Study the drawing (mm; zero at the part's minimum x, y, z) and answer. Coordinates: 2 decimals unless noted, no trailing zeros. Order: outer loops, then holes, each group sorted by start corner. A loop starts at its lowest first (then second) coordinate and runs counter-clockwise, first axis right, second up.
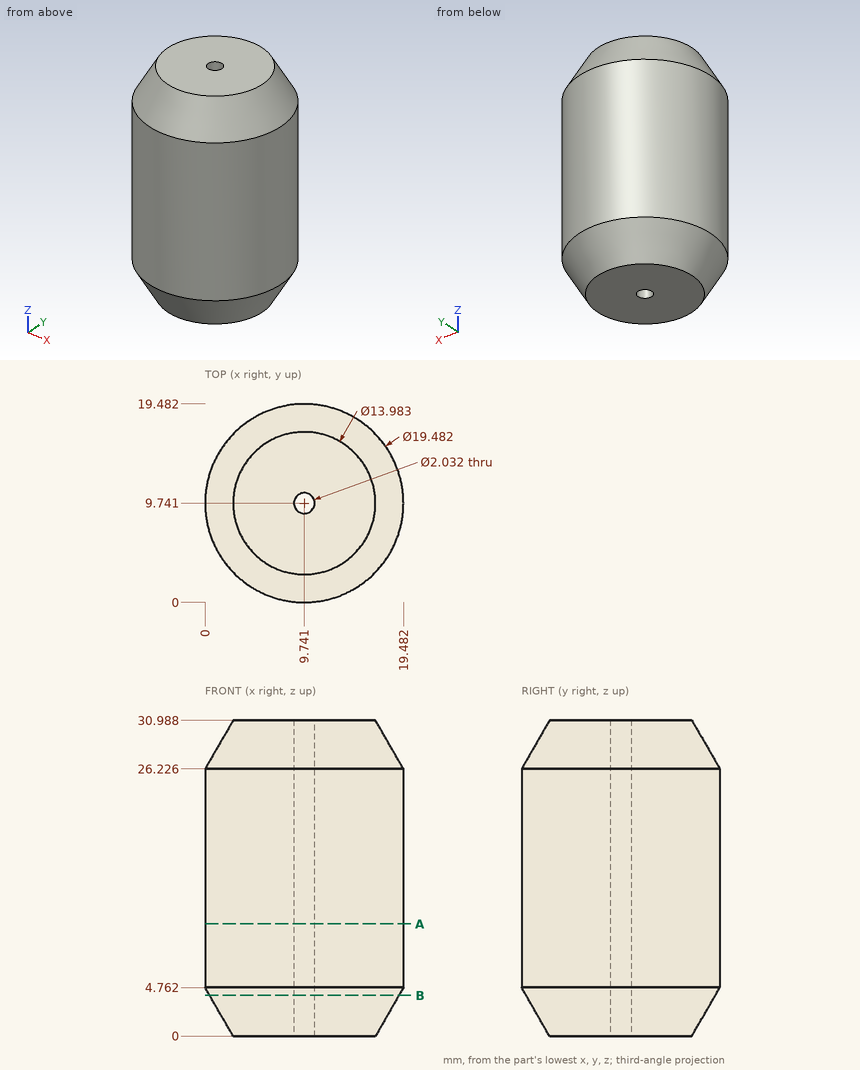
1) Flat-ended cylindrical pins translate along their axes: pin 1 Ø5 at (x, z) = (6.5, 27) entering from +Y; pin 2 Ø5 at (y, z) = (6.5, 8) entering from +X; pin 3 Ø5 at (y, z) = (14, 27.5) entering from -X. Find the tip coordinate at first contact, or state that the pin passes through.
A:
pin 1: stops at y = 19.44
pin 2: stops at x = 19.45
pin 3: stops at x = 0.23
2) A cutting plane is placed at B-B, the plane z = 4. Determine the outline of the cut face in (x, y) (1 decimal).
A:
outline: circle Ø18.6 at (9.7, 9.7); hole circle Ø2 at (9.7, 9.7)
3) Straight lines are drawn through the part: line 1 (Z direction, x = 17.25, y = 10.25) (1 decimal); line 2 (Z direction, x = 6.25, y = 18.25) (1 decimal); line 3 (Y direction, x = 13.75, z = 16.5) (1 decimal). For each, find the intervals that lie inside material, in ascending order.
A:
line 1: z = 0.9 to 30.1
line 2: z = 3.8 to 27.2
line 3: y = 0.9 to 18.6
4) A cutting plane is placed at A-A, the plane z = 11. Determine the outline of the cut face in (x, y) (1 decimal), and give its area (3 significant figures).
A:
outline: circle Ø19.5 at (9.7, 9.7); hole circle Ø2 at (9.7, 9.7)
area: 295 mm2
